Autodesk Inventor part; units mm, degrees
ref_plane "Work Plane1" through (-21, -21, -14) normal (0, 0, 1) x (1, 0, 0)
ref_plane "Work Plane2" through (-21.15, 33.85, -45.625) normal (0, 1, 0) x (0, 0, 1)
ref_plane "YZ Plane" through (0, 0, 0) normal (1, 0, 0) x (0, 1, 0)
sketch "Sketch1" plane through (0, 0, 0) normal (0, 0, 1) x (1, 0, 0)
  line L0 (-20, 16.5858) -> (-16.5858, 20)
  line L1 (-20, -16.5858) -> (-20, 16.5858)
  line L2 (-16.5858, -20) -> (-20, -16.5858)
  line L3 (16.5858, -20) -> (-16.5858, -20)
  line L4 (20, -16.5858) -> (16.5858, -20)
  line L5 (20, 16.5858) -> (20, -16.5858)
  line L6 (16.5858, 20) -> (20, 16.5858)
  line L7 (-16.5858, 20) -> (16.5858, 20)
  circle A0 centre (15.5, -15.5) radius 1.5
  circle A1 centre (-15.5, 15.5) radius 1.5
  circle A2 centre (-15.5, -15.5) radius 1.5
  circle A3 centre (15.5, 15.5) radius 1.5
  circle A4 centre (0, 0) radius 11
  circle A5 centre (0, 0) radius 4.9
  line L8 (13.1931, -21.15) -> (-13.1931, -21.15)
  line L9 (-21.15, -13.1931) -> (-21.15, 13.1931)
  line L10 (21.15, 21.15) -> (-21.15, 21.15)
  line L11 (-21.15, 21.15) -> (-21.15, -21.15)
  line L12 (-21.15, -21.15) -> (21.15, -21.15)
  line L13 (21.15, -21.15) -> (21.15, 21.15)
  line L14 (21.15, 21.15) -> (-21.15, -21.15) construction
  line L15 (-21.15, 21.15) -> (21.15, -21.15) construction
  line L16 (23.15, -23.15) -> (-23.15, -23.15)
  line L17 (-23.15, -23.15) -> (-23.15, 21.15)
  line L18 (23.15, 21.15) -> (23.15, -23.15)
  line L19 (23.15, 21.15) -> (-23.15, 21.15)
  line L20 (-23.15, 21.15) -> (-23.1187, 21.15)
  line L21 (23.15, 21.15) -> (21.15, 21.15)
  line L22 (-13.1931, -21.15) -> (13.1931, -21.15)
  dimension "d0" = 2
extrude "Extrusion1" add sketch "Sketch1" along normal blind 2 contours L0 L7 L6 L5 L4 L3 L2 L1 | L12 L13 L19 L18 L16 L17 L11 L9 L8 | L8 L12 L11 L9 L10 L13
sketch "Sketch2" plane through (0, 0, 0) normal (0, 0, -1) x (-1, 0, 0)
  line L0 (21, -10) -> (21, 10)
  line L1 (-21, 10) -> (-21, -10)
  line L2 (-198.65, 21.15) -> (16.15, 21.15)
  line L3 (21, -21.15) -> (-21, -21.15)
  line L4 (-21, -21.15) -> (-21, 21.15)
  line L5 (-21, 21.15) -> (21, 21.15)
  line L6 (21, 21.15) -> (21, -21.15)
  line L7 (21, -21.15) -> (-21, 21.15) construction
  line L8 (-21, -21.15) -> (21, 21.15) construction
  line L9 (23.15, -23.15) -> (-23.15, -23.15)
  line L10 (-23.15, -23.15) -> (-23.15, 21.15)
  line L11 (23.15, 21.15) -> (23.15, -23.15)
  line L12 (-23.15, 21.15) -> (23.15, 21.15)
  line L13 (21, 21.15) -> (23.15, 21.15)
  line L14 (23.15, 21.15) -> (-21, 21.15)
  line L15 (-21, 21.15) -> (-23.15, 21.15)
  point P0 (0, 0)
ref_plane "Work Plane1" through (-21, -21, -14) normal (0, 0, 1) x (1, 0, 0)
extrude "Extrusion2" add sketch "Sketch2" along normal up to surface (14 mm away) contours L0 L6 L12 L11 L9 L10 L2 L4 L1 L3
sketch "Sketch3" plane through (-23.15, 21.15, 2) normal (0, 1, 0) x (1, 0, 0)
  line L0 (44.15, 2) -> (2.15, 2)
  line L1 (2.15, 2) -> (2.15, 16)
  line L2 (0, 16) -> (2.15, 16)
  line L3 (0, 16) -> (0, 0)
  line L4 (46.3, 0) -> (0, 0)
  line L5 (46.3, 0) -> (46.3, 16)
  line L6 (44.15, 16) -> (46.3, 16)
  line L7 (44.15, 2) -> (44.15, 16)
  arc A0 (2, -201.375) -> (7, -206.375) centre (7, -201.375) ccw
  line L8 (7, -206.375) -> (221.8, -206.375)
  arc A1 (221.8, -206.375) -> (226.8, -201.375) centre (221.8, -201.375) ccw
  line L9 (226.8, -201.375) -> (226.8, -174.375)
  arc A2 (226.8, -174.375) -> (221.8, -169.375) centre (221.8, -174.375) ccw
  line L10 (221.8, -169.375) -> (151.8, -169.375)
  arc A3 (146.8, -164.375) -> (151.8, -169.375) centre (151.8, -164.375) ccw
  line L11 (146.8, -164.375) -> (146.8, 5.625)
  arc A4 (151.8, 10.625) -> (146.8, 5.625) centre (151.8, 5.625) ccw
  line L12 (151.8, 10.625) -> (221.8, 10.625)
  arc A5 (221.8, 10.625) -> (226.8, 15.625) centre (221.8, 15.625) ccw
  line L13 (226.8, 15.625) -> (226.8, 42.625)
  arc A6 (226.8, 42.625) -> (221.8, 47.625) centre (221.8, 42.625) ccw
  line L14 (221.8, 47.625) -> (7, 47.625)
  arc A7 (7, 47.625) -> (2, 42.625) centre (7, 42.625) ccw
  line L15 (2, 42.625) -> (2, 5)
  arc A8 (2, 5) -> (7, 0) centre (7, 5) ccw
  line L16 (7, 0) -> (78.6, 0)
  arc A9 (83.6, -5) -> (78.6, 0) centre (78.6, -5) ccw
  line L17 (83.6, -5) -> (83.6, -153.75)
  arc A10 (78.6, -158.75) -> (83.6, -153.75) centre (78.6, -153.75) ccw
  line L18 (78.6, -158.75) -> (7, -158.75)
  arc A11 (7, -158.75) -> (2, -163.75) centre (7, -163.75) ccw
  line L19 (2, -163.75) -> (2, -201.375)
  line L20 (2, 5) -> (0, 5)
  circle A12 centre (208.3, 29.125) radius 5
  circle A13 centre (208.3, -187.875) radius 5
  circle A14 centre (20.5, 29.125) radius 5
  circle A15 centre (20.5, -187.875) radius 5
  point P0 (23.15, 2)
  point P1 (2, 16)
ref_plane "Work Plane2" through (-21.15, 33.85, -45.625) normal (0, 1, 0) x (0, 0, 1)
extrude "Extrusion3" add sketch "Sketch3" along normal up to surface (12.7 mm away) contours A8 L4 L3 L20 L1 L0 | L0 L1 A8 | L20 L3 L2 L15
sketch "Sketch4" plane through (-23.15, -23.15, -14) normal (-1, 0, 0) x (0, 0, 1)
  line L0 (0, 0) -> (0, 57)
  line L1 (16, 0) -> (16, 57)
  line L2 (0, 57) -> (16, 57)
  line L3 (16, 57) -> (16, 44.5)
  line L4 (16, 44.5) -> (0, 44.5)
  line L5 (0, 44.5) -> (0, 57)
  circle A0 centre (8, 50.75) radius 2.5
  point P0 (14, 23.15)
  dimension "d7" = 12.5
  dimension "d8" = 5
extrude "Extrusion4" cut sketch "Sketch4" against normal blind 2 contours A0
ref_plane "Work Plane3" through (81.25, 21.15, 81.375) normal (0, -1, 0) x (0, 0, 1)
sketch "Sketch5" plane through (81.25, 21.15, 81.375) normal (0, -1, 0) x (0, 0, 1)
  line L0 (-95.375, 58.1) -> (-79.375, 58.1)
  line L1 (-95.375, 58.1) -> (-79.375, 58.1)
  line L2 (-79.375, 104.4) -> (-79.375, 58.1)
  line L3 (-95.375, 104.4) -> (-79.375, 104.4)
  line L4 (-95.375, 58.1) -> (-95.375, 104.4)
  line L5 (-95.375, 58.1) -> (-79.375, 58.1)
  line L6 (-79.375, 58.1) -> (-79.375, 42.1)
  line L7 (-79.375, 42.1) -> (-95.375, 42.1)
  line L8 (-95.375, 42.1) -> (-95.375, 58.1)
  circle A0 centre (-87.375, 50.1) radius 2.5
  point P0 (-81.375, 81.25)
  dimension "d11" = 16
  dimension "d12" = 16
  dimension "d13" = 5
extrude "Extrusion6" add sketch "Sketch5" along normal blind 5 contours L0 L6 L7 L8
sketch "Sketch6" plane through (0, 0, 2) normal (0, 0, 1) x (1, 0, 0)
  circle A0 centre (0, 0) radius 11
  circle A1 centre (15.5, 15.5) radius 1.5
  circle A2 centre (15.5, -15.5) radius 1.5
  circle A3 centre (-15.5, -15.5) radius 1.5
  circle A4 centre (-15.5, 15.5) radius 1.5
  circle A5 centre (0, 0) radius 11.25
  circle A6 centre (15.5, 15.5) radius 1.75
  circle A7 centre (-15.5, 15.5) radius 1.75
  circle A8 centre (15.5, -15.5) radius 1.75
  circle A9 centre (-15.5, -15.5) radius 1.75
  point P0 (0, 0)
  dimension "d18" = 0.25
  dimension "d19" = 0.25
  dimension "d20" = 0.25
  dimension "d21" = 0.25
  dimension "d22" = 0.25
extrude "Extrusion7" cut sketch "Sketch6" against normal up to surface (2 mm away) contours A0 | A1 | A2 | A3 | A4 | A5 | A6 | A7 | A8 | A9
properties part number "PancakeNema17MotorMountOffset"
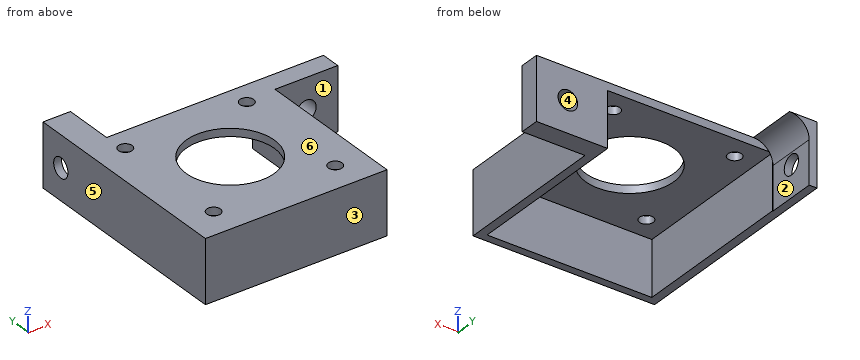
Geometry check sheet. Reference: the model listing, model coordinates, mm. Face numbers are marked on the shaded views. A direction names the side the tool comes from. Round coordinates to 2 decimals unless told otherwise and drop trailing zeros. Order: outer loops, then holes, each group sorted by start corner. A loop starts at its lowest first (then second) coordinate and runs counter-clockwise, first axis right, second up. Notation, with made-up numbers: (33.25, 59) - (50.25, 59) arc R18 ccw to (50.25, 64) - close; hole circle Ø8 at (37, 15). An arc over 180 degrees is marked (long way). Use a Markdown table: item, result. Add a question column.
(1) Sectioned sample at C-C, the plane x = 31.15. Enter the section's corners in (y, z), and give its area (3 significant figures).
(2) Tool access check on the marked faces 1, 2 and 3. Record the directions out of +Z, -Z, +X, -X, +Y, -Y that give a thin tool (end or side, any length) a straight path to the whole face; none if there is none.
(3) Depth check by flat-ended pin: pin 1 (8 mm diameter, centred on y = -12.5, z = -11, fed in from +X); pin 2 (4.5 mm diameter, centred on x = -15.5, y = 15.5, fed in from -Z); pin 3 (8 mm diameter, centred on x = 17.5, z = -8, fed in from +Y); pin 4 (3 mm diameter, centred on x = 31.15, z = -6, fed in from +Y). Enter the tip coordinate at first touch or a pass-through.
(4) Sectioned sample at B-B, the plane y = 27.6. Enter the section's corners in (x, z), and give its area (3 significant figures).
(5) Material ranges on line 1 along X through (y, z) = (18.15, -6); line 2 along Y through (x, z) = (0, 0.6); line 3 along X through (y, z) = (14.5, -11.5), recorded low to high. Write a range as [from, to].
(6) Sectioned sample at D-D, the plane z = -12.75. Enter the section's corners in (x, y), and give its area (3 significant figures).
(7) Release check for a two-part mould opening along Z. For the marked faces 4, 5 and 6 record: pulls with the +Z half, pulls with the -Z half, needs draft (parallel to the pull), parting line crosses it, or undercut.
(8) Sectioned sample at A-A, the plane x = 15.5. Enter the section's corners in (y, z).
Answers below:
| question | item | result |
|---|---|---|
| 1 | outline | (16.15, -14) - (21.15, -14) - (21.15, -8.5) - (16.15, -8.5) - close; (16.15, -3.5) - (21.15, -3.5) - (21.15, 2) - (16.15, 2) - close |
| 1 | area | 55.0 mm² |
| 2 | face 1 | +Z, -Z, +X, -Y |
| 2 | face 2 | -Z, +X, +Y |
| 2 | face 3 | +Z, -Z, +X, -X, -Y |
| 3 | pin 1 | x = 23.15 |
| 3 | pin 2 | z = 0 |
| 3 | pin 3 | y = 21.15 |
| 3 | pin 4 | through |
| 4 | outline | (-23.15, -14) - (-21.15, -14) - (-21.15, -8.5) - (-23.15, -8.5) - close; (-23.15, -3.5) - (-21.15, -3.5) - (-21.15, -3) arc R5 cw to (-16.15, 2) - (-23.15, 2) - close |
| 4 | area | 27.4 mm² |
| 5 | line 1 | [-23.15, -21], [21, 28.65], [33.65, 39.15] |
| 5 | line 2 | [-23.15, -11.25], [11.25, 21.15] |
| 5 | line 3 | [-23.15, -21], [21, 23.15] |
| 6 | outline | (-23.15, -23.15) - (23.15, -23.15) - (23.15, 16.15) - (39.15, 16.15) - (39.15, 21.15) - (21, 21.15) - (21, -21.15) - (-21, -21.15) - (-21, 21.15) - (-21.15, 21.15) - (-21.15, 33.85) - (-23.15, 33.85) - close |
| 6 | area | 380 mm² |
| 7 | face 4 | undercut |
| 7 | face 5 | needs draft |
| 7 | face 6 | pulls with the +Z half |
| 8 | outline | (-23.15, -14) - (-21.15, -14) - (-21.15, 0) - (-17.25, 0) - (-17.25, 2) - (-23.15, 2) - close; (-13.75, 0) - (13.75, 0) - (13.75, 2) - (-13.75, 2) - close; (17.25, 0) - (21.15, 0) - (21.15, 2) - (17.25, 2) - close |
